Answer from the drawing. Dimensions are ordinates in mm from the lowest x, y and z of the part. A direction names the side the tool comes from. Round coordinates to 2 decimals unless told otherwise and drop trailing zeros. Order: outer loops, then holes, each group sorted by start corner. A loop starts at its lowest first (then second) coordinate and runs counter-clockwise, first axis right, second up.
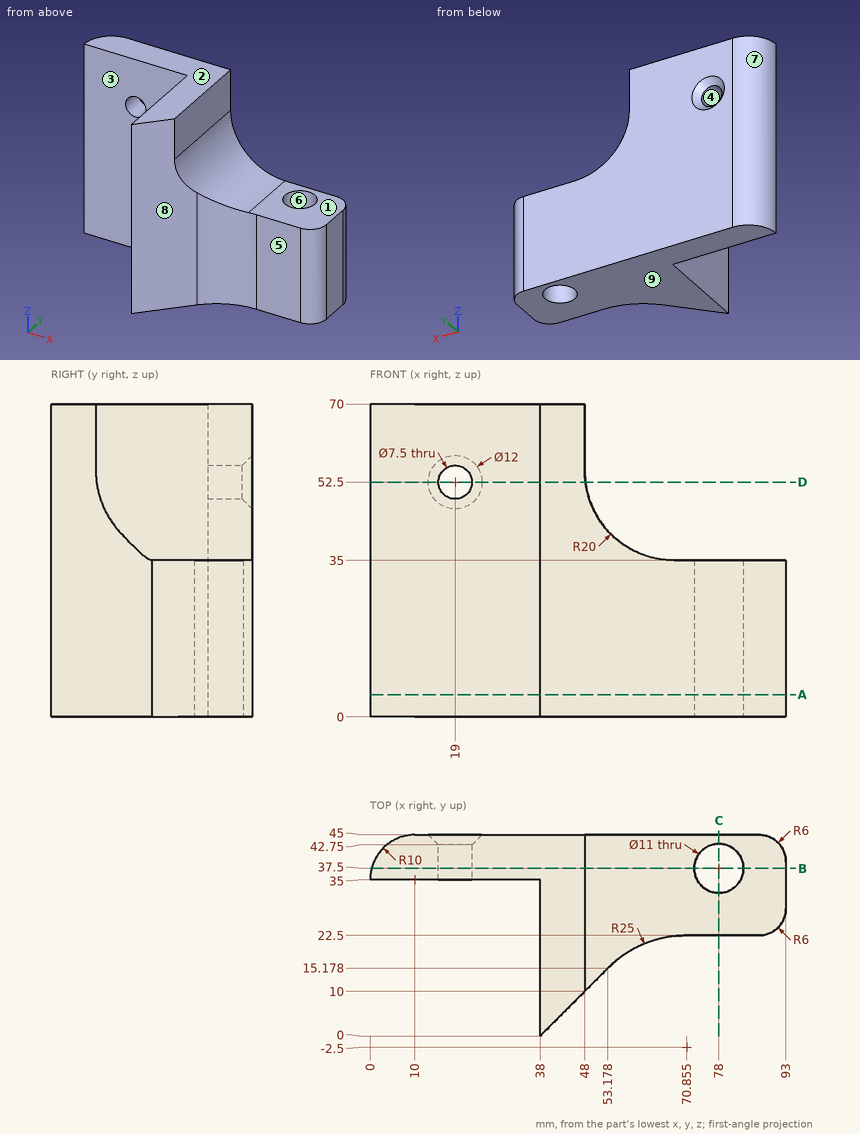
Q1. For a pull along Y with two mould halves and no side action, classify the marked faces 6, 7, 8 and 9 as released by +Y, released by -Y, zero draft, split by the parting line, or undercut.
Outcome:
face 6: undercut
face 7: released by +Y
face 8: released by -Y
face 9: zero draft
Q2. A cutting plane is placed at C-C, the plane x = 78. Give the vertices of the cut face in (y, z).
Outcome:
outline: (22.5, 0) - (32, 0) - (32, 35) - (22.5, 35) - close; (43, 0) - (45, 0) - (45, 35) - (43, 35) - close
Q3. A cutting plane is placed at A-A, the plane z = 5. Give the vertices of the cut face in (x, y) (1 decimal).
Outcome:
outline: (0, 35) - (38, 35) - (38, 0) - (53.2, 15.2) arc R25 cw to (70.9, 22.5) - (87, 22.5) arc R6 ccw to (93, 28.5) - (93, 39) arc R6 ccw to (87, 45) - (10, 45) arc R10 ccw to start; hole circle Ø11 at (78, 37.5)
Q4. A cutting plane is placed at D-D, the plane z = 52.5. Give the vertices of the cut face in (x, y), plus the area to 3 significant figures.
Outcome:
outline: (0, 35) - (15.25, 35) - (15.25, 42.75) - (13, 45) - (10, 45) arc R10 ccw to start; (22.75, 35) - (38, 35) - (38, 0) - (48.16, 10.16) - (48.16, 45) - (25, 45) - (22.75, 42.75) - close
area: 684 mm2
Q5. Flat-ended cylindrical pins translate along their axes: pin 1 (12 mm diameter, centred on x = 20, z = 19, fed in from -Y); pin 2 (10.5 mm diameter, centred on y = 22.5, z = 18.5, fed in from -X); pin 3 (11.5 mm diameter, centred on x = 79.5, y = 39, fed in from +Z). Find the tip coordinate at first contact, or state that the pin passes through.
Outcome:
pin 1: stops at y = 35
pin 2: stops at x = 38
pin 3: stops at z = 35
Q6. Straight lines are drawn through the part: probe 1 along Y at (x, z) = (78, 26); probe 2 along Z at (x, y) = (19, 37.5); probe 3 along X at (y, z) = (30, 31). For each, find the intervals that lie inside material, in ascending order.
Outcome:
probe 1: y = 22.5 to 32, 43 to 45
probe 2: z = 0 to 48.75, 56.25 to 70
probe 3: x = 38 to 93
Q7. For the marked faces 1, 2, 3, 4 and 5, determine the directions among +Z, -Z, +X, -X, +Y, -Y from which every point of the face is accessible in a straight line to the end or side of a thin tool.
Outcome:
face 1: +Z, +X, +Y, -Y
face 2: +Z, +X, -X, +Y, -Y
face 3: +Z, -Z, -X, -Y
face 4: +Y, -Y
face 5: +Z, -Z, +X, -Y
Q8. A cutting plane is placed at B-B, the plane y = 37.5. Give the vertices of the cut face in (x, z), plus the area to 3 significant figures.
Outcome:
outline: (0.32, 0) - (72.5, 0) - (72.5, 35) - (68, 35) arc R20 cw to (48, 55) - (48, 70) - (0.32, 70) - close; (83.5, 0) - (93, 0) - (93, 35) - (83.5, 35) - close; hole circle Ø7.5 at (19, 52.5)
area: 4,570 mm2
